Solid Edge part; units mm, degrees
sketch "Sketch1" plane through (0, 0, 0) normal (0, -1, 0) x (1, 0, 0)
  line L0 (20, 36) -> (-16, 36)
  line L1 (-16, 36) -> (-16, -36)
  line L2 (-16, -36) -> (20, -36)
  line L3 (20, -36) -> (20, -40)
  line L4 (20, -40) -> (-20, -40)
  line L5 (-20, -40) -> (-20, 40)
  line L6 (-20, 40) -> (20, 40)
  line L7 (20, 40) -> (20, 36)
  dimension "D1" = 20
  dimension "D2" = 20
  dimension "D3" = 20
extrude "Protrusion1" add sketch "Sketch1" against normal blind 350
sketch "Sketch2" plane through (0, 175, 40) normal (0, 0, 1) x (0, 1, 0)
  line L0 (-175, 20) -> (-135, -20)
extrude "Cutout1" cut sketch "Sketch2" against normal through all material side at (0.0354, 19.9646, 40)
sketch "Sketch3" plane through (0, 175, 40) normal (0, 0, 1) x (0, 1, 0)
  line L0 (175, 20) -> (135, -20)
extrude "Cutout2" cut sketch "Sketch3" against normal through all material side at (0.0354, 330.0354, 40)
hole "Bohrung_1" at (-16, 142.5, 17) direction (-1, 0, 0) diameter 6 end up to next
hole "Hole1" at (-16, 207.5, 17) direction (-1, 0, 0) diameter 6 end up to next
hole "Bohrung_3" at (-16, 50, 15.6) direction (-1, 0, 0) diameter 5 end up to next
hole "Hole2" at (-16, 105, 15.6) direction (-1, 0, 0) diameter 5 end up to next
hole "Hole3" at (-16, 245, 15.6) direction (-1, 0, 0) diameter 5 end up to next
hole "Hole4" at (-16, 300, 15.6) direction (-1, 0, 0) diameter 5 end up to next
properties material "AlMgSi 0,5-1"
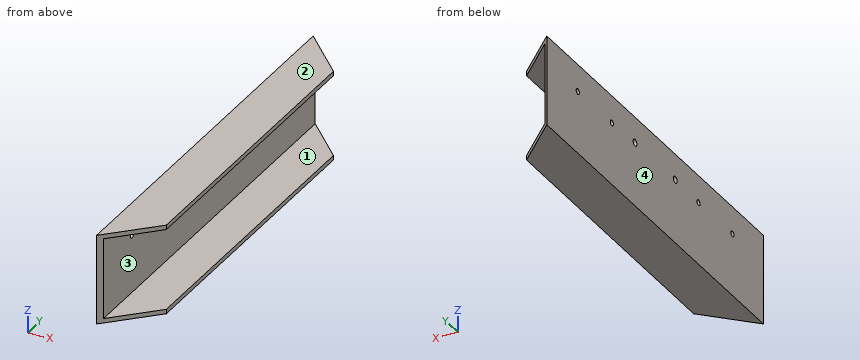
Geometry check sheet. Reference: the model listing, model coordinates, mm. Face numbers are marked on the shaded views. Give positions to 0.01 mm unless a question says otherwise; leave off trailing zeros. Order: outer loops, then holes, each group sorted by start corner. A loop starts at its lowest first (then second) coordinate and runs counter-clockwise, first axis right, second up.
1) Cross-section at B-B (y = 142.5). Record the boundary of the cut face in (x, z), then the cut area to 3 significant figures.
Results are:
outline: (-20, -40) - (20, -40) - (20, -36) - (-16, -36) - (-16, 14) - (-20, 14) - close; (-20, 20) - (-16, 20) - (-16, 36) - (20, 36) - (20, 40) - (-20, 40) - close
area: 584 mm2
2) Cross-section at D-D (y = 70). Record the boundary of the cut face in (x, z), then the cut area to 3 significant figures.
Results are:
outline: (-20, -40) - (20, -40) - (20, -36) - (-16, -36) - (-16, 36) - (20, 36) - (20, 40) - (-20, 40) - close
area: 608 mm2
3) Cross-section at A-A (x = 13). Record the boundary of the cut face in (y, z).
Results are:
outline: (33, -40) - (317, -40) - (317, -36) - (33, -36) - close; (33, 36) - (317, 36) - (317, 40) - (33, 40) - close
4) Cross-section at C-C (x = -1.5). Record the boundary of the cut face in (y, z).
Results are:
outline: (18.5, -40) - (331.5, -40) - (331.5, -36) - (18.5, -36) - close; (18.5, 36) - (331.5, 36) - (331.5, 40) - (18.5, 40) - close
5) Draft check along Z on the marked faces 1, 2, 3 and 4. Enter one of: released by +Z, released by -Z, zero draft, split by the parting line, or undercut.
Results are:
face 1: undercut
face 2: released by +Z
face 3: undercut
face 4: zero draft
6) Material ranges on probe 1 along Z at (x, y) = (-5, 178); probe 2 along Z at (x, y) = (-18, 207); probe 3 along X at (y, z) = (112, -5.5), recorded low to high.
Results are:
probe 1: z = -40 to -36, 36 to 40
probe 2: z = -40 to 14.04, 19.96 to 40
probe 3: x = -20 to -16
7) Gauge pin test, flat ends, axial feed: pin 1 (8 mm diameter, centred on y = 50, z = 15.6, fed in from +X); pin 2 (3 mm diameter, centred on y = 300, z = 15.6, fed in from -X). Record the tip position at first contact, or that the pin passes through.
Results are:
pin 1: stops at x = -16
pin 2: passes through
